Geometry: final body of the model. Coordinates: model frame, mm. Round coordinates to 2 decimals unless told otherwise and drop trailing zeros. Loops run counter-clockwise (first coordinate to the right, second up) from the corner with the lowest first, then second, coordinate; pieces in that order, holes last. Notation, with made-up numbers: M 41.5,66 L 83.5,66 A22 ccw 83.5,98 Z; hole C 52,50.5 d3. An arc over 180 degrees is marked long. Answer as a JSON object with one key per item and string values.
```python
from build123d import *

# Parameters (mm, degrees)
F0_W     = 50.8
F0_H     = 69.85
F1_DEPTH = 3.175
F3_D     = 6.5278
F5_D     = 3.15
F7_D     = 12.7


with BuildPart() as f1:
    # F0 (on Front) → F1 (new body)
    with BuildSketch(Plane.XZ):
        Rectangle(F0_W, F0_H)
    extrude(amount=F1_DEPTH)

    # F3 (through all)
    with Locations(Plane.XZ.offset(3.175)):
        with Locations((-12.7, 22.225), (12.7, 22.225)):
            Hole(F3_D / 2)

    # F5 (through all)
    with Locations(Plane.XZ.offset(3.175)):
        with Locations((-8.9454650708, -0.381), (8.9454650708, -0.381), (17.8909301416, -15.875), (8.9454650708, -31.369), (-8.9454650708, -31.369), (-17.8909301416, -15.875)):
            Hole(F5_D / 2)

    # F7 (through all)
    with Locations(Plane.XZ.offset(3.175)):
        with Locations((0, -10.9855)):
            Hole(F7_D / 2)


solid = f1.part
```
1) Cut plane C-C on y = -2.2. Count the separate pieces of the cut face and the enclosed holes in it, and give its area (3 significant figures).
Geometry results:
{"separate pieces": "1", "enclosed holes": "9", "area": "3,310 mm2"}
2) Cut plane B-B on x = 0. Return the cut outline in (y, z) (1 decimal), and give its area (3 significant figures).
Geometry results:
{"outline": "M -3.2,-34.9 L 0,-34.9 L 0,-17.3 L -3.2,-17.3 Z; M -3.2,-4.6 L 0,-4.6 L 0,34.9 L -3.2,34.9 Z", "area": "181 mm2"}
3) Pull-direction query (Z, two-part tool) for faces 1 (the face through (0, -2, -34.925)), 2 (the face through (-10.294, -1.565, 24.431)), 3 (the face through (0, 0, 0)); classes: +Z half, -Z half, draft (parallel to the pull), parting line (faces both ways), or undercut.
Geometry results:
{"face 1": "-Z half", "face 2": "undercut", "face 3": "draft"}
4) First-contact query: pin 1 (3 mm diameter, centred on x = -8.95, z = -31.37, fed in from -Y); pin 2 (4 mm diameter, centred on x = 8.95, z = -31.37, fed in from +Y). Flat tips, straight axial feed; report the tip coordinate or a pass-through.
Geometry results:
{"pin 1": "through", "pin 2": "y = 0"}
5) Line query: probe 1 along X at (y, z) = (-1.15, -31.5) (3 decimals); probe 2 along Z at (x, y) = (18, -1.9) (3 decimals); probe 3 along Z at (x, y) = (12.7, -0.85) (3 decimals). Output: solid intervals per line, ascending.
Geometry results:
{"probe 1": "-25.4 to -10.515, -7.376 to 7.376, 10.515 to 25.4", "probe 2": "-34.925 to -17.446, -14.304 to 34.925", "probe 3": "-34.925 to 18.961, 25.489 to 34.925"}
6) Cut plane A-A on x = -12.7. Return the cut outline in (y, z) (3 decimals).
Geometry results:
{"outline": "M -3.175,-34.925 L 0,-34.925 L 0,18.961 L -3.175,18.961 Z; M -3.175,25.489 L 0,25.489 L 0,34.925 L -3.175,34.925 Z"}
